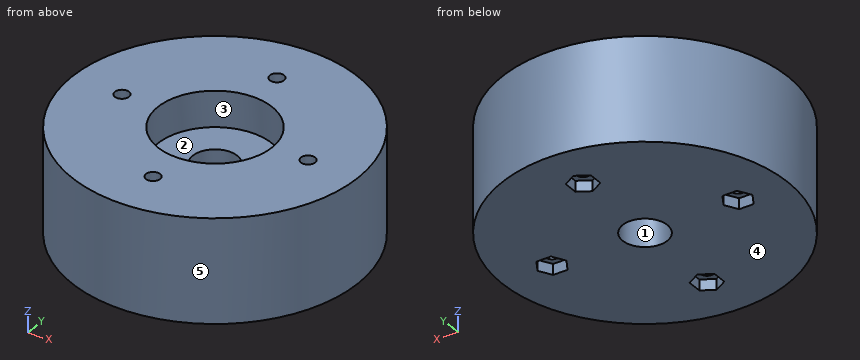
Autodesk Inventor part; units mm, degrees
ref_plane "YZ Plane" through (0, 0, 0) normal (1, 0, 0) x (0, 1, 0)
ref_plane "XZ Plane" through (0, 0, 0) normal (0, 1, 0) x (-1, 0, 0)
ref_plane "XY Plane" through (0, 0, 0) normal (0, 0, 1) x (1, 0, 0)
sketch "Esquisse1" plane through (0, 0, 0) normal (0, 0, 1) x (1, 0, 0)
  circle A0 centre (0, 0) radius 40
  circle A1 centre (0, 0) radius 6.25
  line L0 (0, 0) -> (16.25, 0) construction
  circle A2 centre (0, 0) radius 16.25 construction
  line L1 (6.25, 0) -> (16.25, 0) construction
  line L2 (0, 0) -> (0, 26) construction
  circle A3 centre (0, 26) radius 2
  circle A4 centre (-26, 0) radius 2
  circle A5 centre (0, -26) radius 2
  circle A6 centre (26, 0) radius 2
  dimension "d1" = 12.5
  dimension "d0" = 80
  dimension "d3" = 10
  dimension "d5" = 4
  dimension "d6" = 26
  dimension "d9" = 360
extrude "Extrusion1" add sketch "Esquisse1" along normal blind 29
sketch "Esquisse2" plane through (0, 0, 29) normal (0, 0, 1) x (1, 0, 0)
  circle A0 centre (0, 0) radius 6.25
  circle A1 centre (0, 0) radius 40
  circle A2 centre (0, 0) radius 16
  line L0 (0, 0) -> (-16, 0) construction
  dimension "d41" = 16
extrude "Extrusion2" cut sketch "Esquisse2" against normal blind 10 contours A2
sketch "Esquisse3" plane through (0, 0, 0) normal (0, 0, -1) x (-1, 0, 0)
  circle A0 centre (0, 0) radius 6.25
  circle A1 centre (-26, 0) radius 2
  circle A2 centre (0, -26) radius 2
  circle A3 centre (26, 0) radius 2
  circle A4 centre (0, 26) radius 2
  circle A5 centre (0, 0) radius 40
  line L0 (3.5, 23.9793) -> (0, 21.9585)
  line L1 (0, 21.9585) -> (-3.5, 23.9793)
  line L2 (-3.5, 23.9793) -> (-3.5, 28.0207)
  line L3 (-3.5, 28.0207) -> (0, 30.0415)
  line L4 (0, 30.0415) -> (3.5, 28.0207)
  line L5 (3.5, 28.0207) -> (3.5, 23.9793)
  line L6 (-3.5, 23.9793) -> (3.5, 23.9793) construction
  line L7 (0, 0) -> (0, -40) construction
  line L8 (-23.9793, 3.5) -> (-21.9585, 0)
  line L9 (-21.9585, 0) -> (-23.9793, -3.5)
  line L10 (-23.9793, -3.5) -> (-28.0207, -3.5)
  line L11 (-28.0207, -3.5) -> (-30.0415, 0)
  line L12 (-30.0415, 0) -> (-28.0207, 3.5)
  line L13 (-28.0207, 3.5) -> (-23.9793, 3.5)
  line L14 (-3.5, -23.9793) -> (0, -21.9585)
  line L15 (0, -21.9585) -> (3.5, -23.9793)
  line L16 (3.5, -23.9793) -> (3.5, -28.0207)
  line L17 (3.5, -28.0207) -> (0, -30.0415)
  line L18 (0, -30.0415) -> (-3.5, -28.0207)
  line L19 (-3.5, -28.0207) -> (-3.5, -23.9793)
  line L20 (23.9793, -3.5) -> (21.9585, 0)
  line L21 (21.9585, 0) -> (23.9793, 3.5)
  line L22 (23.9793, 3.5) -> (28.0207, 3.5)
  line L23 (28.0207, 3.5) -> (30.0415, 0)
  line L24 (30.0415, 0) -> (28.0207, -3.5)
  line L25 (28.0207, -3.5) -> (23.9793, -3.5)
  point P0 (-23.9793, 3.5)
  point P1 (-3.5, -23.9793)
  point P2 (23.9793, -3.5)
  dimension "d18" = 7
  dimension "d21" = 360
extrude "Extrusion3" cut sketch "Esquisse3" against normal blind 3 contours L0 L1 L2 L3 L4 L5 | L8 L9 L10 L11 L12 L13 | L14 L15 L16 L17 L18 L19 | L20 L21 L22 L23 L24 L25
properties part number "bowl_v2"
Check sheet for the modelled part. Datum: model origin and axes. Units: mm. Face numbers are marked on the shaded views. A direction names the side the tool comes from. Coordinates: 2 decimals unless noted, no trailing zeros. Write each loop counter-clockwise with the first axis right and the second up, starting at its lowest first coordinate (ties: lowest second). Pieces come first, ordered by that corner, then holes. Notation, with made-up numbers: M 10.5,44 L 62.5,44 A28 cw 62.5,72 Z; hole C -30.75,22 d11. An arc over 180 degrees is marked long. Answer as CSV lines item,"result".
Q1. Mould release check, pull along X, two halves, no side actions. Record for the marked faces 3, 4 and 5: released by +X, released by -X, zero draft, split by the parting line, or undercut.
Check result:
face 3,"undercut"
face 4,"zero draft"
face 5,"split by the parting line"
Q2. Material ranges on probe 1 along Y at (x, z) = (0, 21.5); probe 2 along Y at (x, z) = (0, 12); probe 3 along Z at (x, y) = (12, 4.5), recorded low to high. Write a range as from..to.
Check result:
probe 1,"-40..-28, -24..-16, 16..24, 28..40"
probe 2,"-40..-28, -24..-6.25, 6.25..24, 28..40"
probe 3,"0..19"
Q3. Cross-section at A-A (z = 2). Record the boundary of the cut face in (x, y).
Check result:
outline,"C 0,0 d80; hole M -30.04,0 L -28.02,-3.5 L -23.98,-3.5 L -21.96,0 L -23.98,3.5 L -28.02,3.5 Z; hole C 0,0 d12.5; hole M -3.5,-28.02 L 0,-30.04 L 3.5,-28.02 L 3.5,-23.98 L 0,-21.96 L -3.5,-23.98 Z; hole M -3.5,23.98 L 0,21.96 L 3.5,23.98 L 3.5,28.02 L 0,30.04 L -3.5,28.02 Z; hole M 21.96,0 L 23.98,-3.5 L 28.02,-3.5 L 30.04,0 L 28.02,3.5 L 23.98,3.5 Z"
Q4. Cross-section at D-D (x = -7.5). Record the boundary of the cut face in (y, z), then the cut area to 3 significant figures.
Check result:
outline,"M -39.29,0 L 39.29,0 L 39.29,29 L 14.13,29 L 14.13,19 L -14.13,19 L -14.13,29 L -39.29,29 Z"
area,"2,000 mm^2"
Q5. Set-up check for the marked faces 1 and 2: record each of +Z, -Z, +X, -X, +Y, -Y from which the full face is reachable in a straight line by a thin tool's end or side.
Check result:
face 1,"+Z, -Z"
face 2,"+Z"
Q6. Cross-section at B-B (y = -27). Record the boundary of the cut face in (x, z), then the cut area to 3 significant figures.
Check result:
outline,"M -29.51,0 L -3.5,0 L -3.5,3 L -1.73,3 L -1.73,29 L -29.51,29 Z; M 1.73,3 L 3.5,3 L 3.5,0 L 29.51,0 L 29.51,29 L 1.73,29 Z"
area,"1,600 mm^2"
Q7. Cross-section at C-C (x = -25.5). Record the boundary of the cut face in (y, z).
Check result:
outline,"M -30.82,0 L -3.5,0 L -3.5,3 L -1.94,3 L -1.94,29 L -30.82,29 Z; M 1.94,3 L 3.5,3 L 3.5,0 L 30.82,0 L 30.82,29 L 1.94,29 Z"
Q8. Go/stop test with flat-tipped pins: pin 1 (8 mm diameter, centred on y = -18, z = 5, fed in from +X); pin 2 (0.9 mm diameter, centred on y = -27, z = 1.5, fed in from -X); pin 3 (2.5 mm diameter, centred on x = -27, z = 1.5, fed in from +Y); pin 4 (10 mm diameter, centred on x = 0, y = 0, fed in from +Z). Record where each tip stops, or that it passes through.
Check result:
pin 1,"x = 37.47"
pin 2,"x = -29.92"
pin 3,"y = 30.61"
pin 4,"through"
